Check sheet for the modelled part. Datum: model origin and axes. Units: mm. Coordinates: 2 decimals unless noted, no trailing zeros. Write each loop counter-clockwise with the first axis right and the second up, starting at its lowest first coordinate (ties: lowest second). Pieces come first, ordered by that corner, then holes. Notation, with made-up numbers: (-35.5, 87) -> (-2.5, 87) arc R26 cw to (-2.5, 112) -> close; hole circle Ø3 at (73, 29). An arc over 180 degrees is marked (long way). One line per item, written item: value. Start each with the question number.
1) Sectioned sample at A-A on z = 4. Enter the section's corners in (x, y).
2) Scan lines: line 1 along Z through (x, y) = (-47.5, -4); line 2 along Y through (x, z) = (20, 4.75); line 3 along X through (y, z) = (-0.25, 6). Record each from-to range of solid material in increasing order. Write a range as [from, to].
3) Sectioned sample at B-B on x = -53.5. Enter the section's corners in (y, z), plus the area to 3 significant figures.
4) Sectioned sample at C-C on y = 6.5. Enter the section's corners in (x, z).
Autodesk Inventor part; units mm, degrees
ref_plane "YZ Plane" through (0, 0, 0) normal (1, 0, 0) x (0, 1, 0)
ref_plane "XZ Plane" through (0, 0, 0) normal (0, 1, 0) x (-1, 0, 0)
ref_plane "XY Plane" through (0, 0, 0) normal (0, 0, 1) x (1, 0, 0)
sketch "Skizze1" plane through (0, 0, 0) normal (0, 0, 1) x (1, 0, 0)
  line L0 (-74.0778, 7.5) -> (-74.0778, -7.5)
  line L1 (-74.0778, -7.5) -> (5.9222, -7.5)
  line L2 (6.251, -7.4728) -> (39.251, -1.9728)
  line L3 (39.251, 1.9728) -> (6.251, 7.4728)
  line L4 (5.9222, 7.5) -> (-74.0778, 7.5)
  arc A0 (6.251, 7.4728) -> (5.9222, 7.5) centre (5.9222, 5.5) ccw
  arc A1 (5.9222, -7.5) -> (6.251, -7.4728) centre (5.9222, -5.5) ccw
  arc A2 (39.251, -1.9728) -> (39.251, 1.9728) centre (38.9222, 0) ccw
  line L5 (-97.0778, 0) -> (63.9222, 0)
  point P0 (0, 0)
  dimension "d0" = 2
  dimension "d1" = 2
  dimension "d2" = 115
  dimension "d3" = 80
  dimension "d9" = 15
extrude "Extrusion1" add sketch "Skizze1" along normal blind 5
sketch "Skizze2" plane through (0, 0, 5) normal (0, 0, 1) x (1, 0, 0)
  arc A0 (39.251, -1.9728) -> (39.251, 1.9728) centre (38.9222, 0) ccw
  circle A1 centre (38.9222, 0) radius 1.25
  point P0 (0, 0)
  dimension "d6" = 2.5
extrude "Extrusion2" add sketch "Skizze2" along normal blind 3 draft -10
properties part number "Sensor"
Answers:
1. outline: (-74.08, -7.5) -> (5.92, -7.5) arc R2 ccw to (6.25, -7.47) -> (39.25, -1.97) arc R2 ccw to (39.25, 1.97) -> (6.25, 7.47) arc R2 ccw to (5.92, 7.5) -> (-74.08, 7.5) -> close
2. line 1: z = [0, 5]
2. line 2: y = [-5.18, 5.18]
2. line 3: x = [37.88, 39.97]
3. outline: (-7.5, 0) -> (7.5, 0) -> (7.5, 5) -> (-7.5, 5) -> close
3. area: 75.0 mm2
4. outline: (-74.08, 0) -> (12.09, 0) -> (12.09, 5) -> (-74.08, 5) -> close
